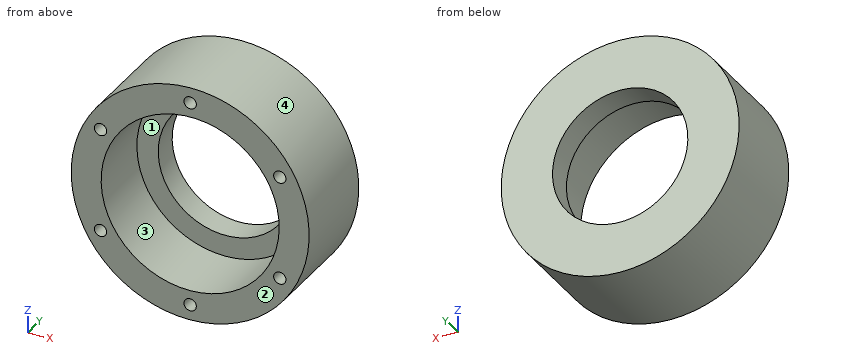
from build123d import *

# Parameters (mm, degrees)
SKETCH2_R          = 29
EXTRUDE1_DEPTH     = 23
SKETCH3_R          = 21.7
CUT_EXTRUDE1_DEPTH = 16.55
SKETCH4_R          = 16.5
CUT_EXTRUDE2_DEPTH = 48.021271782
CUT_EXTRUDE3_START = -3
SKETCH5_R          = 1.5
CUT_EXTRUDE3_DEPTH = 45.021271782


with BuildPart() as part:
    # Sketch2 → Extrude1 (new body)
    with BuildSketch(Plane(origin=(0, 0, 0), x_dir=(1, 0, 0), z_dir=(0, 1, 0))):
        with Locations(Location((0, 0, 0), (0, 0, 270))):
            Circle(SKETCH2_R)
    extrude(amount=EXTRUDE1_DEPTH)

    # Sketch3 → Cut-Extrude1 (cut)
    with BuildSketch(Plane.XZ):
        with Locations(Location((0, 0, 0), (0, 0, 270))):
            Circle(SKETCH3_R)
    extrude(amount=-CUT_EXTRUDE1_DEPTH, mode=Mode.SUBTRACT)

    # Sketch4 → Cut-Extrude2 (cut, through all)
    with BuildSketch(Plane(origin=(0, 23, 0), x_dir=(1, 0, 0), z_dir=(0, 1, 0))):
        with Locations(Location((0, 0, 0), (0, 0, 270))):
            Circle(SKETCH4_R)
    extrude(amount=-CUT_EXTRUDE2_DEPTH, mode=Mode.SUBTRACT)

    # Sketch5 → Cut-Extrude3 (cut, through all)
    with BuildSketch(Plane(origin=(0, 23, 0), x_dir=(1, 0, 0), z_dir=(0, 1, 0)).offset(CUT_EXTRUDE3_START)):
        with Locations(Location((0, 25.230472928, 0), (0, 0, 270))):
            Circle(SKETCH5_R)
        with Locations(Location((21.850230505, 12.615236464, 0), (0, 0, 270))):
            Circle(SKETCH5_R)
        with Locations(Location((21.850230505, -12.615236464, 0), (0, 0, 270))):
            Circle(SKETCH5_R)
        with Locations(Location((0, -25.230472928, 0), (0, 0, 270))):
            Circle(SKETCH5_R)
        with Locations(Location((-21.850230505, -12.615236464, 0), (0, 0, 270))):
            Circle(SKETCH5_R)
        with Locations(Location((-21.850230505, 12.615236464, 0), (0, 0, 270))):
            Circle(SKETCH5_R)
    extrude(amount=-CUT_EXTRUDE3_DEPTH, mode=Mode.SUBTRACT)


solid = part.part
Input: part model. Units: mm. Frame: model coordinates. Face numbers are marked on the shaded views. Coordinates: 2 decimals unless noted, no trailing zeros. Write each loop counter-clockwise with the first axis right and the second up, starting at its lowest first coordinate (ties: lowest second). Pieces come first, ordered by that corner, then holes. Notation, with made-up numbers: M 58.5,61.25 L 72.5,61.25 A22 cw 72.5,82.25 Z; hole C -7.5,60 d5. An arc over 180 degrees is marked long. Answer as a JSON object with one key per item and string values. Group by question number.
(1) Section C-C on y = 18.75. Output: boundary loops of the cut face in (x, z).
(2) Contact query for flat-ended pins moving along their axis: P1, Ø10, axis at y = 15.5, z = -1, coming from the +X side; P2, Ø1, axis at x = -8.5, y = 15, coming from the -Z side; P3, Ø2.5, axis at x = -21.85, z = -12.62, coming from the -Y side. Output: stop coordinate, or through.
(3) Section A-A on x = 0. Output: boundary loops of the cut face in (y, z).
(4) Section D-D on x = 8. Output: boundary loops of the cut face in (y, z), plus the area to 3 significant figures.
(5) Ray query, line 1 along X through (y, z) = (8.5, 0); line 2 along X through (y, z) = (19.75, 0); line 3 along X through (y, z) = (19.5, 12). Return the intervals inside material, ascending. Write a range as [from, to].
(6) Section B-B on z = 0. Output: boundary loops of the cut face in (x, y), plus the area to 3 significant figures.
(7) Mould query, pull axis X, two halves, no side actions, for the marked faces 1, 2, 3 and 4. Classes: pulls with the +X half, pulls with the -X half, needs draft (parallel to the pull), parting line crosses it, or undercut.
Result set:
{
 "1": {"outline": "C 0,0 d58; hole C -21.85,-12.62 d3; hole C -21.85,12.62 d3; hole C 0,0 d33; hole C 0,-25.23 d3; hole C 0,25.23 d3; hole C 21.85,-12.62 d3; hole C 21.85,12.62 d3"},
 "2": {"P1": "stops at x = 29", "P2": "stops at z = -27.87", "P3": "stops at y = 20"},
 "3": {"outline": "M 0,-29 L 23,-29 L 23,-16.5 L 16.55,-16.5 L 16.55,-21.7 L 0,-21.7 L 0,-23.73 L 20,-23.73 L 20,-26.73 L 0,-26.73 Z; M 0,21.7 L 16.55,21.7 L 16.55,16.5 L 23,16.5 L 23,29 L 0,29 L 0,26.73 L 20,26.73 L 20,23.73 L 0,23.73 Z"},
 "4": {"outline": "M 0,-27.87 L 23,-27.87 L 23,-14.43 L 16.55,-14.43 L 16.55,-20.17 L 0,-20.17 Z; M 0,20.17 L 16.55,20.17 L 16.55,14.43 L 23,14.43 L 23,27.87 L 0,27.87 Z", "area": "428 mm2"},
 "5": {"line 1": "x = [-29, -21.7], [21.7, 29]", "line 2": "x = [-29, -16.5], [16.5, 29]", "line 3": "x = [-26.4, -23.22], [-20.48, -11.32], [11.32, 20.48], [23.22, 26.4]"},
 "6": {"outline": "M -29,0 L -21.7,0 L -21.7,16.55 L -16.5,16.55 L -16.5,23 L -29,23 Z; M 16.5,16.55 L 21.7,16.55 L 21.7,0 L 29,0 L 29,23 L 16.5,23 Z", "area": "403 mm2"},
 "7": {"face 1": "undercut", "face 2": "needs draft", "face 3": "undercut", "face 4": "parting line crosses it"}
}
